Source: CAD feature listing. Evaluate the final solid. Frame: model axes, mm. A direction names the side the tool comes from. Give positions to 0.01 mm unless a question says otherwise; leave off trailing zeros. Order: outer loops, then holes, each group sorted by start corner. A loop starts at its lowest first (then second) coordinate and runs counter-clockwise, first axis right, second up.
1) First-contact query: P1, Ø12, axis at x = 5, z = -110, coming from the +Y side; P2, Ø4, axis at x = -37, y = -51, coming from the +Z side; P3, Ø0.6, axis at x = -31.5, z = 233, coming from the +Y side. Flat tips, straight axial feed; report the tip coordinate or a pass-through.
2) Draft query along X for faces 1 (the face through (95.745, -49.516, 233.514)), 2 (the face through (-144.5, -48, 3)), 3 (the face through (-95.745, -50.484, 233.514)). Return one class per face: released by +X, released by -X, zero draft, split by the parting line, or undercut.
3) Section B-B, the plane z = -14. Return loops of the section in (x, y).
4) Section A-A, the plane x = 56. Return loops of the section in (y, z), plus the area to 4 significant figures.
5) Access query for faces 4 (the face through (-2, -100, -3)), 5 (the face through (-2, -48, -229.5)), 6 (the face through (-2, -27, 232.5)). Directions: +Z, -Z, +X, -X, +Y, -Y. A direction counts if a zero-diameter tool reaches every point of the face in a straight line with its end or side. Return the directions, or none.
6) Section D-D, the plane y = -50. Return loops of the section in (x, z), plus the area to 3 significant figures.
7) Section C-C, the plane y = -22. Return loops of the section in (x, z).
8) Material intervals for line 1 (X direction, y = -16, z = -13.5); line 2 (Z direction, x = -90.5, y = -31.5); line 3 (Z direction, x = -55, y = -31), sorted ascending.
```python
from build123d import *

# Parameters (mm, degrees)
SKETCH2_W           = 295
SKETCH2_H           = 465
BOSS_EXTRUDE1_DEPTH = 100
SHELL5_T            = -3
CUT_EXTRUDE5_DEPTH  = 462
BOSS_EXTRUDE2_START = 2
BOSS_EXTRUDE2_DEPTH = 2


with BuildPart() as part:
    # Sketch2 → Boss-Extrude1 (new body)
    with BuildSketch(Plane(origin=(0, 0, 0), x_dir=(1, 0, 0), z_dir=(0, 1, 0))):
        Rectangle(SKETCH2_W, SKETCH2_H)
    extrude(amount=-BOSS_EXTRUDE1_DEPTH)

    # Shell5
    shell5_openings = [part.faces().sort_by_distance(p)[0] for p in [
        (0, 0, 0),
    ]]
    offset(amount=SHELL5_T, openings=shell5_openings, kind=Kind.INTERSECTION)

    # Sketch3 → Cut-Extrude5 (cut)
    with BuildSketch(Plane.XY.offset(232.5)):
        with BuildLine():
            Line((-73.75, -35), (73.75, -35))
            ThreePointArc((73.75, -35), (88.75, -50), (73.75, -65))
            Line((73.75, -65), (-73.75, -65))
            ThreePointArc((-73.75, -65), (-88.75, -50), (-73.75, -35))
        make_face()
    extrude(amount=-CUT_EXTRUDE5_DEPTH, mode=Mode.SUBTRACT)

    # Sketch3<4> → Boss-Extrude2 (add)
    with BuildSketch(Plane.XY.offset(232.5).offset(BOSS_EXTRUDE2_START)):
        with BuildLine():
            Line((-73.75, -28), (73.75, -28))
            ThreePointArc((73.75, -28), (95.75, -50), (73.75, -72))
            Line((73.75, -72), (-73.75, -72))
            ThreePointArc((-73.75, -72), (-95.75, -50), (-73.75, -28))
        make_face()
        with BuildLine():
            Line((-73.75, -35), (73.75, -35))
            ThreePointArc((73.75, -35), (88.75, -50), (73.75, -65))
            Line((73.75, -65), (-73.75, -65))
            ThreePointArc((-73.75, -65), (-88.75, -50), (-73.75, -35))
        make_face(mode=Mode.SUBTRACT)
    extrude(amount=-BOSS_EXTRUDE2_DEPTH)


solid = part.part
```
From the geometry:
1. P1: stops at y = -97
1. P2: stops at z = -229.5
1. P3: stops at y = -28
2. face 1: released by +X
2. face 2: undercut
2. face 3: released by -X
3. outline: (-147.5, -100) - (147.5, -100) - (147.5, 0) - (144.5, 0) - (144.5, -97) - (-144.5, -97) - (-144.5, 0) - (-147.5, 0) - close
4. outline: (-100, -232.5) - (0, -232.5) - (0, -229.5) - (-97, -229.5) - (-97, 229.5) - (-65, 229.5) - (-65, 234.5) - (-72, 234.5) - (-72, 232.5) - (-100, 232.5) - close; (-35, 229.5) - (0, 229.5) - (0, 232.5) - (-28, 232.5) - (-28, 234.5) - (-35, 234.5) - close
4. area: 1,915 mm2
5. face 4: +Z, -Z, +X, -X, -Y
5. face 5: +Y
5. face 6: +Z
6. outline: (-147.5, -232.5) - (147.5, -232.5) - (147.5, 232.5) - (95.75, 232.5) - (95.75, 234.5) - (88.75, 234.5) - (88.75, 229.5) - (144.5, 229.5) - (144.5, -229.5) - (-144.5, -229.5) - (-144.5, 229.5) - (-88.75, 229.5) - (-88.75, 234.5) - (-95.75, 234.5) - (-95.75, 232.5) - (-147.5, 232.5) - close
6. area: 4,020 mm2
7. outline: (-147.5, -232.5) - (147.5, -232.5) - (147.5, 232.5) - (-147.5, 232.5) - close; hole (-144.5, -229.5) - (144.5, -229.5) - (144.5, 229.5) - (-144.5, 229.5) - close
8. line 1: x = -147.5 to -144.5, 144.5 to 147.5
8. line 2: z = -232.5 to -229.5, 229.5 to 232.5
8. line 3: z = -232.5 to -229.5, 229.5 to 234.5
